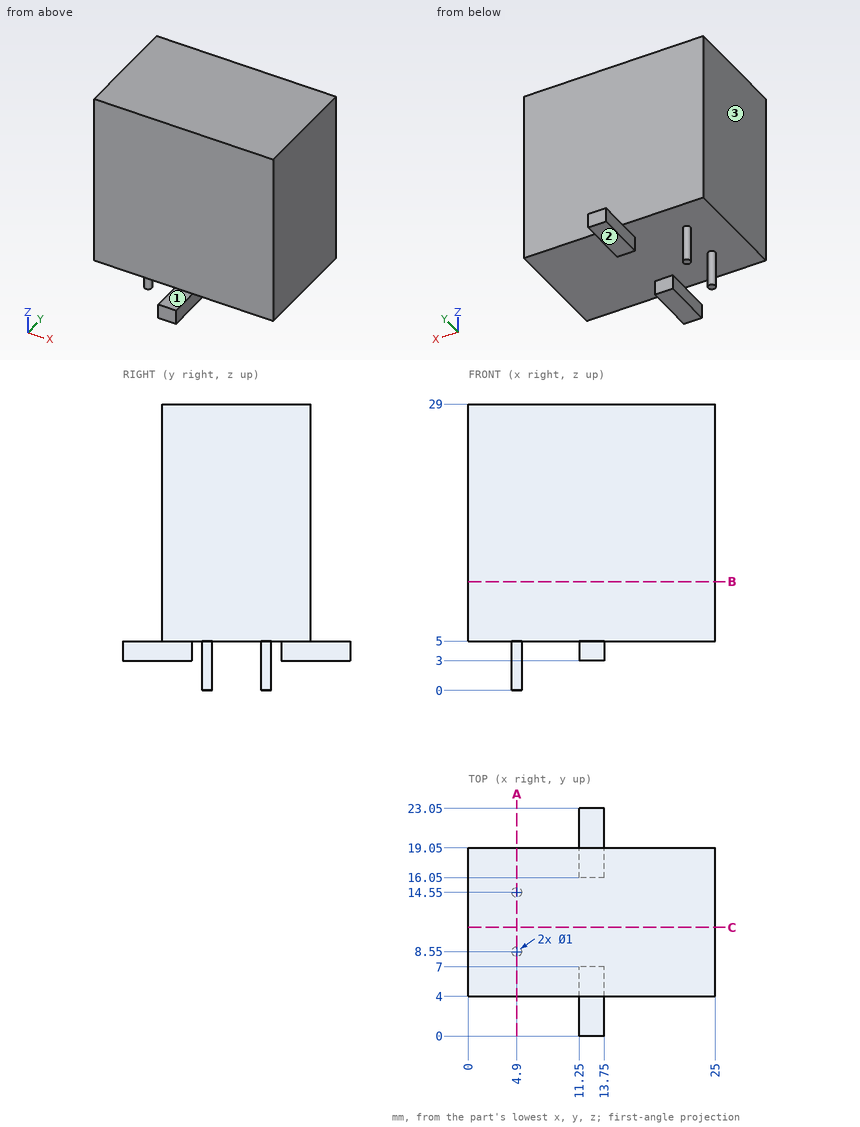
Drawing for the job (mm, zero at the part's lowest x, y, z). Round coordinates to 2 decimals unless told otherwise and drop trailing zeros. Order: outer loops, then holes, each group sorted by start corner. A loop starts at its lowest first (then second) coordinate and runs counter-clockwise, first axis right, second up.
Item 1: Probe line 1 along Y through (x, z) = (12.25, 4); line 2 along Y through (x, z) = (17.5, 12); line 3 along Z through (x, y) = (18.75, 6). List the from-to ranges inside material, lowest first.
Item 2: Mould opens along Z. For the marked faces 1, 2 and 3 say: pulls with the +Z half, pulls with the -Z half, needs draft (parallel to the pull), parting line crosses it, or undercut.
Item 3: Pin check, flat tips, straight feed: pin 1 (4 mm diameter, centred on x = 8.5, z = 21.5, fed in from -Y); pin 2 (0.6 mm diameter, centred on y = 3, z = 4, fed in from -X); pin 3 (2 mm diameter, centred on x = 12, y = 1.5, fed in from +Z). Stop position of each tip, or through.
Item 4: Saw through at C-C on y = 11. Write the cut outline in (x, z).
Item 5: Saw through at B-B on z = 11. Write the cut outline in (x, y).
Item 6: Saw through at A-A on x = 4.9. Write the cut outline in (y, z).
Reported:
1. line 1: y = 0 to 7, 16.05 to 23.05
1. line 2: y = 4 to 19.05
1. line 3: z = 5 to 29
2. face 1: pulls with the +Z half
2. face 2: pulls with the -Z half
2. face 3: needs draft
3. pin 1: stops at y = 4
3. pin 2: stops at x = 11.25
3. pin 3: stops at z = 5
4. outline: (0, 5) - (25, 5) - (25, 29) - (0, 29) - close
5. outline: (0, 4) - (25, 4) - (25, 19.05) - (0, 19.05) - close
6. outline: (4, 5) - (8.05, 5) - (8.05, 0) - (9.05, 0) - (9.05, 5) - (14.05, 5) - (14.05, 0) - (15.05, 0) - (15.05, 5) - (19.05, 5) - (19.05, 29) - (4, 29) - close
